from build123d import *

# Parameters (mm, degrees)
SKETCH1_W           = 17
SKETCH1_H           = 17
BOSS_EXTRUDE1_DEPTH = 249.5
SKETCH2_W           = 12
SKETCH2_H           = 45
CUT_EXTRUDE1_DEPTH  = 252.098088404
CUT_EXTRUDE2_DEPTH  = 252.098088404


with BuildPart() as part:
    # Sketch1 → Boss-Extrude1 (new body)
    with BuildSketch(Plane(origin=(0, 0, 0), x_dir=(1, 0, 0), z_dir=(0, 1, 0))):
        with BuildLine():
            Line((0.5, 0), (19.5, 0))
            ThreePointArc((19.5, 0), (19.853553391, 0.146446609), (20, 0.5))
            Line((20, 0.5), (20, 19.5))
            ThreePointArc((20, 19.5), (19.853553391, 19.853553391), (19.5, 20))
            Line((19.5, 20), (0.5, 20))
            ThreePointArc((0.5, 20), (0.146446609, 19.853553391), (0, 19.5))
            Line((0, 19.5), (0, 0.5))
            ThreePointArc((0, 0.5), (0.146446609, 0.146446609), (0.5, 0))
        make_face()
        with Locations((10, 10)):
            Rectangle(SKETCH1_W, SKETCH1_H, mode=Mode.SUBTRACT)
    extrude(amount=BOSS_EXTRUDE1_DEPTH)

    # Sketch2 → Cut-Extrude1 (cut, through all)
    with BuildSketch(Plane.ZY):
        with Locations((-10, 22.5)):
            Rectangle(SKETCH2_W, SKETCH2_H)
        with Locations((-10, 227)):
            Rectangle(SKETCH2_W, SKETCH2_H)
    extrude(amount=-CUT_EXTRUDE1_DEPTH, mode=Mode.SUBTRACT)

    # Sketch3 → Cut-Extrude2 (cut, through all)
    with BuildSketch(Plane(origin=(0, 0, -20), x_dir=(-1, 0, 0), z_dir=(0, 0, -1))):
        Polygon((0, 235.5), (-3, 235.5), (-17, 249.5), (0, 249.5), align=None)
        Polygon((-17, 0), (0, 0), (0, 14), (-3, 14), align=None)
    extrude(amount=-CUT_EXTRUDE2_DEPTH, mode=Mode.SUBTRACT)


solid = part.part
Here's how the part is built. I have some questions about the finished solid (model axes, mm). A direction names the side the tool comes from. Give positions to 0.01 mm unless a question says otherwise; leave off trailing zeros. Order: outer loops, then holes, each group sorted by start corner. A loop starts at its lowest first (then second) coordinate and runs counter-clockwise, first axis right, second up. Notation, with made-up numbers: (-14.75, 16) -> (5.25, 16) arc R9 ccw to (5.25, 20) -> close; hole circle Ø5 at (40, 9.25). An arc over 180 degrees is marked (long way). One line per item, written item: value. Start each with the question number.
1. Imagine slicing it at A-A, the plane z = -10. List the corners of the cut face in (x, y) for me, plus the area to 4 significant figures.
2. Imagine slicing it at B-B, the plane x = 13.75. List the corners of the cut face in (y, z) for me, plus the area to 3 significant figures.
3. We'd pull the mould along X, two halves only. Please class faces 3 (the face through (20, 123, -10)), 4 (the face through (10, 123, 0)), 5 (the face through (10, 123, -1.5)): released by +X, released by -X, zero draft, split by the parting line, or undercut.
4. Will these pins go through, and if not, where does the flat tip stop? pin 1 Ø0.8 at (x, z) = (19, -8.5) entering from +Y; pin 2 Ø1.2 at (x, z) = (19, -10) entering from -Y; pin 3 Ø12 at (x, z) = (9, -2.5) entering from +Y; pin 4 Ø0.9 at (x, z) = (2, -17.5) entering from -Y.
5. I need wall thicknesses on probe 1 along X at (y, z) = (139, -13); probe 2 along Z at (x, y) = (9.25, 166); probe 3 along Y at (x, z) = (19, -7.5). Which ranges of each line are inside material? Lowest first, please. Write a range as from..to.
6. Imagine slicing it at C-C, the plane y = 188.5. List the corners of the cut face in (x, z) for me, plus the area to 3 significant figures.
7. For faces 1 (the face through (10, 123, -18.5)), 2 (the face through (9.9, 242.4, -19.3)), which set-ups out of +Z, -Z, +X, -X, +Y, -Y let a thin tool reach every point of the face, with its end or its side?
8. Imagine slicing it at D-D, the plane y = 40.5. List the corners of the cut face in (x, z) for me, plus the area to 3 significant figures.
Values follow:
1. outline: (0, 45) -> (1.5, 45) -> (1.5, 204.5) -> (0, 204.5) -> close; (18.5, 45) -> (20, 45) -> (20, 204.5) -> (18.5, 204.5) -> close
1. area: 478.5 mm2
2. outline: (3.25, -20) -> (246.25, -20) -> (246.25, -18.5) -> (3.25, -18.5) -> close; (3.25, -1.5) -> (246.25, -1.5) -> (246.25, 0) -> (3.25, 0) -> close
2. area: 729 mm2
3. face 3: released by +X
3. face 4: zero draft
3. face 5: undercut
4. pin 1: stops at y = 204.5
4. pin 2: stops at y = 45
4. pin 3: stops at y = 247.42
4. pin 4: passes through
5. probe 1: x = 0..1.5, 18.5..20
5. probe 2: z = -20..-18.5, -1.5..0
5. probe 3: y = 45..204.5
6. outline: (0, -19.5) arc R0.5 ccw to (0.5, -20) -> (19.5, -20) arc R0.5 ccw to (20, -19.5) -> (20, -0.5) arc R0.5 ccw to (19.5, 0) -> (0.5, 0) arc R0.5 ccw to (0, -0.5) -> close; hole (1.5, -18.5) -> (18.5, -18.5) -> (18.5, -1.5) -> (1.5, -1.5) -> close
6. area: 111 mm2
7. face 1: +Y, -Y
7. face 2: +Z, -Z, -X, +Y
8. outline: (0, -19.5) arc R0.5 ccw to (0.5, -20) -> (19.5, -20) arc R0.5 ccw to (20, -19.5) -> (20, -16) -> (18.5, -16) -> (18.5, -18.5) -> (1.5, -18.5) -> (1.5, -16) -> (0, -16) -> close; (0, -4) -> (1.5, -4) -> (1.5, -1.5) -> (18.5, -1.5) -> (18.5, -4) -> (20, -4) -> (20, -0.5) arc R0.5 ccw to (19.5, 0) -> (0.5, 0) arc R0.5 ccw to (0, -0.5) -> close
8. area: 74.8 mm2
